```python
from build123d import *

# Parameters (mm, degrees)
SKETCH_5_R               = 4
EXTRUDE_3_DEPTH          = 42
CUT_EXTRUDE_2_DEPTH      = 47.113989348
CUT_EXTRUDE_2_DEPTH_BACK = 47.113989348
EXTRUDE_4_DEPTH          = 12
EXTRUDE_4_DEPTH_BACK     = 12
SKETCH_7_R               = 2.5


with BuildPart() as part:
    # Эскиз4 → Повернуть1 (revolve)
    with BuildSketch(Plane.XY, mode=Mode.PRIVATE) as revolve_1_sk:
        Polygon((-16.5, 0), (-16.5, 9.5), (-6.8, 9.5), (-6.8, 8), (-6, 8), (-6, 9.5), (6, 9.5), (6, 8), (6.8, 8), (6.8, 9.5), (16.5, 9.5), (16.5, 0), align=None)
    revolve(revolve_1_sk.sketch.rotate(Axis((-16.5, 0, 0), (1, 0, 0)), 180), axis=Axis((-16.5, 0, 0), (1, 0, 0)))

    # Эскиз5 → Бобышка-Вытянуть3 (add)
    with BuildSketch(Plane(origin=(0, 0, 0), x_dir=(1, 0, 0), z_dir=(0, 1, 0))):
        with Locations(Location((-12, 0, 0), (0, 0, 270))):
            Circle(SKETCH_5_R)
        with Locations(Location((12, 0, 0), (0, 0, 270))):
            Circle(SKETCH_5_R)
    extrude(amount=-EXTRUDE_3_DEPTH)

    # Эскиз6 → Вырез-Вытянуть2 (cut, two sides: drawn at the far end of the back side and taken through both)
    with BuildSketch(Plane(origin=(0, 0, 0), x_dir=(0, 0, -1), z_dir=(1, 0, 0)).offset(-CUT_EXTRUDE_2_DEPTH_BACK)):
        Polygon((4, -42), (-4, -35.971567599), (-4, -42), align=None)
    extrude(amount=CUT_EXTRUDE_2_DEPTH + CUT_EXTRUDE_2_DEPTH_BACK, mode=Mode.SUBTRACT)

    # Эскиз7 → Бобышка-Вытянуть4 (add, two sides: drawn at the far end of the back side and taken through both)
    with BuildSketch(Plane(origin=(0, 0, 0), x_dir=(0, 0, -1), z_dir=(1, 0, 0)).offset(-EXTRUDE_4_DEPTH_BACK)):
        with Locations((0, -22)):
            Circle(SKETCH_7_R)
    extrude(amount=EXTRUDE_4_DEPTH + EXTRUDE_4_DEPTH_BACK)

    # Эскиз8 → Повернуть2 (revolve)
    with BuildSketch(Plane.XY, mode=Mode.PRIVATE) as revolve_2_sk:
        Polygon((-5.5, -22), (-5.5, -16.5), (-3.5, -16.5), (-3.5, -15.5), (3.5, -15.5), (3.5, -16.5), (5.5, -16.5), (5.5, -22), align=None)
    revolve(revolve_2_sk.sketch.rotate(Axis((-20.226487352, -22, 0), (1, 0, 0)), 90), axis=Axis((-20.226487352, -22, 0), (1, 0, 0)))


solid = part.part
```
Check sheet for the modelled part. Datum: model origin and axes. Units: mm. A direction names the side the tool comes from. Coordinates: 2 decimals unless noted, no trailing zeros. Loops run counter-clockwise (first coordinate to the right, second up) from the corner with the lowest first, then second, coordinate; pieces in that order, holes last.
1) Sectioned sample at B-B (x = -2). Record the boundary of the cut face in (y, z).
2) Release check for a two-part mould opening along Y. For faces 3 (the face through (-6.837, -21.249, -2.385)), 4 (the face through (-12.06, -39.03, -0.06)), 5 (the face through (16.5, 0, 0)) record: released by +Y, released by -Y, zero draft, split by the parting line, or undercut.
3) Sectioned sample at C-C (y = -6.5). Record the boundary of the cut face in (x, z).
4) Access from +Z, -Z, +X, -X, +Y, -Y to the whole of each face (thin tool, end or side, straight path). Record for faces 1 (the face through (6.79, -21.249, -2.385)), 2 (the face through (11.94, -39.03, -0.06)).
5) Sectioned sample at A-A (y = -22). Record the boundary of the cut face in (x, z), and give its area (3 significant figures).
6) Sectioned sample at D-D (x = -13). Record the boundary of the cut face in (y, z).
7) Material ranges on probe 1 along X at (y, z) = (-3.5, -7.5); probe 2 along Y at (x, z) = (-2.5, -0.25); probe 3 along X at (y, z) = (-13, -3), recorded low to high.
8) Gauge pin test, flat ends, axial feed: pin 1 (6 mm diameter, centred on x = -6, z = -5.5, fed in from +Y); pin 2 (5 mm diameter, centred on x = 7, z = 2, fed in from -Y); pin 3 (1 mm diameter, centred on x = 2, z = 4, fed in from -Y). Record the tip position at first contact, or that the pin passes through.
Check sheet entries:
1. outline: circle Ø13 at (-22, 0); circle Ø19 at (0, 0)
2. face 3: undercut
2. face 4: released by -Y
2. face 5: zero draft
3. outline: (-16.5, -6.93) - (-6.8, -6.93) - (-6.8, -4.66) - (-6, -4.66) - (-6, -6.93) - (6, -6.93) - (6, -4.66) - (6.8, -4.66) - (6.8, -6.93) - (16.5, -6.93) - (16.5, 6.93) - (6.8, 6.93) - (6.8, 4.66) - (6, 4.66) - (6, 6.93) - (-6, 6.93) - (-6, 4.66) - (-6.8, 4.66) - (-6.8, 6.93) - (-16.5, 6.93) - close
4. face 1: none
4. face 2: +Z, +X, -X, -Y
5. outline: (-8.88, -2.5) - (-5.5, -2.5) - (-5.5, -5.5) - (-3.5, -5.5) - (-3.5, -6.5) - (3.5, -6.5) - (3.5, -5.5) - (5.5, -5.5) - (5.5, -2.5) - (8.88, -2.5) arc R4 ccw (long way) to (8.88, 2.5) - (5.5, 2.5) - (5.5, 5.5) - (3.5, 5.5) - (3.5, 6.5) - (-3.5, 6.5) - (-3.5, 5.5) - (-5.5, 5.5) - (-5.5, 2.5) - (-8.88, 2.5) arc R4 ccw (long way) to start
5. area: 263 mm2
6. outline: (-41.9, -3.87) - (-8.67, -3.87) arc R9.5 ccw (long way) to (-8.67, 3.87) - (-36.07, 3.87) - close
7. probe 1: x = -16.5 to -6.8, -6 to 6, 6.8 to 16.5
7. probe 2: y = -28.5 to -15.5, -9.5 to 9.5
7. probe 3: x = -14.65 to -9.35, 9.35 to 14.65
8. pin 1: stops at y = 9.17
8. pin 2: stops at y = -39.2
8. pin 3: stops at y = -27.48
